Could you check a few things on this model? Use its own coordinates, in mm. Face numbers are marked on the shaded views. A direction names the side the tool comes from. Give positions to 0.01 mm unless a question says otherwise; leave off trailing zeros. Loops run counter-clockwise (first coordinate to the right, second up) from the corner with the lowest first, then second, coordinate; pieces in that order, holes last. Notation, with made-up numbers: M -9,-15.75 L -4,-15.75 A34 cw -4,14.25 Z; hole C 68,-30 d5. An arc over 180 degrees is marked long. Return JSON: item names as keys, results as strings. Group by question number.
1. If we section it at D-D (x = -11.5): Write out the boundary of the cut face in (y, z), plus the area to 3 significant figures.
2. Please list where these lines run through material, in increasing order: line 1 (X direction, y = 58, z = 0); line 2 (Z direction, x = -7, y = 56); line 3 (Y direction, x = 3, z = -9).
3. If we section it at C-C (y = 29.5): Write out the boundary of the cut face in (x, z).
4. For the marked faces 1, 2 and 3, which set-ups out of +Z, -Z, +X, -X, +Y, -Y let a thin tool reach every point of the face, with its end or its side?
5. For pin 1 (5 mm diameter, centred on x = -7.75, z = 13.42, fed in from +Y); pin 2 (5 mm diameter, centred on y = 32, z = 9.5, fed in from +X); pin 3 (0.9 mm diameter, centred on x = 15, z = -0.5, fed in from +Y), each with a flat end and sliding along its axis, tell me the tip position at first contact or that it passes through.
6. If we section it at B-B (z = 0): Write out the boundary of the cut face in (x, y), plus the area to 3 significant figures.
7. If we section it at A-A (x = 0): Write out the boundary of the cut face in (y, z), plus the area to 3 significant figures.
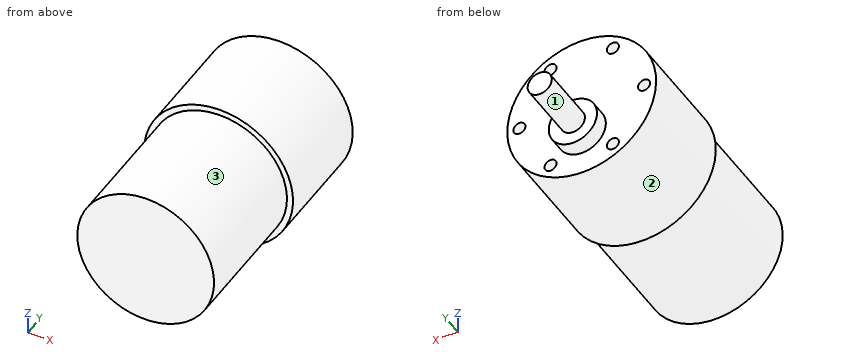
```python
from build123d import *

# Parameters (mm, degrees)
SKETCH_1_R          = 17
EXTRUDE_1_DEPTH     = 33
SKETCH_2_R          = 18.5
EXTRUDE_2_DEPTH     = 27
SKETCH_3_R          = 6
EXTRUDE_3_DEPTH     = 4
SKETCH_4_R          = 3
EXTRUDE_5_DEPTH     = 15
SKETCH_6_R          = 1.5
CUT_EXTRUDE_1_DEPTH = 5


with BuildPart() as part:
    # 草图1 → 凸台-拉伸1 (new body)
    with BuildSketch(Plane(origin=(0, 0, 0), x_dir=(1, 0, 0), z_dir=(0, 1, 0))):
        with Locations(Location((0, 0, 0), (0, 0, 270))):
            Circle(SKETCH_1_R)
    extrude(amount=EXTRUDE_1_DEPTH)

    # 草图2 → 凸台-拉伸2 (add)
    with BuildSketch(Plane(origin=(0, 33, 0), x_dir=(1, 0, 0), z_dir=(0, 1, 0))):
        with Locations(Location((0, 0, 0), (0, 0, 270))):
            Circle(SKETCH_2_R)
    extrude(amount=EXTRUDE_2_DEPTH)

    # 草图3 → 凸台-拉伸3 (add)
    with BuildSketch(Plane(origin=(0, 60, 0), x_dir=(1, 0, 0), z_dir=(0, 1, 0))):
        with Locations(Location((0, 7, 0), (0, 0, 270))):
            Circle(SKETCH_3_R)
    extrude(amount=EXTRUDE_3_DEPTH)

    # 草图4 → 凸台-拉伸5 (add)
    with BuildSketch(Plane(origin=(0, 64, 0), x_dir=(1, 0, 0), z_dir=(0, 1, 0))):
        with Locations(Location((0, 7, 0), (0, 0, 270))):
            Circle(SKETCH_4_R)
    extrude(amount=EXTRUDE_5_DEPTH)

    # 草图6 → 切除-拉伸1 (cut)
    with BuildSketch(Plane(origin=(0, 60, 0), x_dir=(1, 0, 0), z_dir=(0, 1, 0))):
        with Locations(Location((7.75, 13.423393759, 0), (0, 0, 270))):
            Circle(SKETCH_6_R)
        with Locations(Location((15.5, 0, 0), (0, 0, 270))):
            Circle(SKETCH_6_R)
        with Locations(Location((7.75, -13.423393759, 0), (0, 0, 270))):
            Circle(SKETCH_6_R)
        with Locations(Location((-7.75, -13.423393759, 0), (0, 0, 270))):
            Circle(SKETCH_6_R)
        with Locations(Location((-15.5, 0, 0), (0, 0, 270))):
            Circle(SKETCH_6_R)
        with Locations(Location((-7.75, 13.423393759, 0), (0, 0, 270))):
            Circle(SKETCH_6_R)
    extrude(amount=-CUT_EXTRUDE_1_DEPTH, mode=Mode.SUBTRACT)


solid = part.part
```
Answer:
{
 "1": {"outline": "M 0,-12.52 L 33,-12.52 L 33,-14.49 L 60,-14.49 L 60,14.49 L 33,14.49 L 33,12.52 L 0,12.52 Z", "area": "1,610 mm²"},
 "2": {"line 1": "x = -18.5 to -17, -14 to 14, 17 to 18.5", "line 2": "z = -17.12 to -14.72, -12.12 to 12.12, 14.72 to 17.12", "line 3": "y = 0 to 64"},
 "3": {"outline": "C 0,0 d34"},
 "4": {"face 1": "+Y", "face 2": "+Y, -Y", "face 3": "-Y"},
 "5": {"pin 1": "stops at y = 60", "pin 2": "stops at x = 17.04", "pin 3": "stops at y = 55"},
 "6": {"outline": "M -18.5,33 L -17,33 L -17,0 L 17,0 L 17,33 L 18.5,33 L 18.5,60 L 17,60 L 17,55 L 14,55 L 14,60 L -14,60 L -14,55 L -17,55 L -17,60 L -18.5,60 Z", "area": "2,090 mm²"},
 "7": {"outline": "M 0,-17 L 33,-17 L 33,-18.5 L 60,-18.5 L 60,-13 L 64,-13 L 64,-10 L 79,-10 L 79,-4 L 64,-4 L 64,-1 L 60,-1 L 60,18.5 L 33,18.5 L 33,17 L 0,17 Z", "area": "2,260 mm²"}
}
